Check sheet for the modelled part. Datum: model origin and axes. Units: mm. A direction names the side the tool comes from. Round coordinates to 2 decimals unless told otherwise and drop trailing zeros. Write each loop counter-clockwise with the first axis right and the second up, starting at its lowest first coordinate (ties: lowest second). Pieces come first, ordered by that corner, then holes.
Item 1: Go/stop test with flat-tipped pins: pin 1 Ø1.3 at (x, z) = (15, 39.48) entering from -Y; pin 2 Ø12 at (x, z) = (34, 28.5) entering from -Y. Record where each tip stops, or that it passes through.
Item 2: Cross-section at A-A on z = 34. Enter the section's corners in (x, y) (3 decimals), plus the area to 3 significant figures.
Item 3: Release check for a two-part mould opening along Z. For faces 5 (the flat face through (32, -3, 2.5)), 6 (the cylindrical face through (42.526, -7.986, 8.852)), 7 (the cylindrical face through (15, -8, 32)), 8 (the flat face through (49.845, -6, 39)) record: +Z half, -Z half, draft (parallel to the pull), parting line (faces both ways), or undercut.
Item 4: Cross-section at D-D on z = 16. Enter the section's corners in (x, y) (3 decimals).
Item 5: Cross-section at C-C on y = -6. Count the separate pieces of the cut face and the enclosed holes in it, plus the area to 3 significant figures.
Item 6: Material ranges on line 1 (Z direction, x = 15, y = -2.75); line 2 (Z direction, x = 37.86, y = -3.75); line 3 (Z direction, x = 30, y = -6), recorded low to high.
Item 7: Tool access check on faces 1 (the flat face through (30, -7, 41)), 2 (the flat face through (23.08, -5, 56)), 3 (the flat face through (15, -9, 6)), 4 (the cylindrical face through (39.246, -1.232, 69.065)). Record the directions out of +Z, -Z, +X, -X, +Y, -Y that give a thin tool (end or side, any length) a straight path to the whole face; none if there is none.
Item 8: Cross-section at B-B on x = 30.5. Enter the section's corners in (y, z).
from build123d import *

# Parameters (mm, degrees)
SKETCH003_W     = 45
SKETCH003_H     = 75
PAD001_DEPTH    = 7
SKETCH004_R     = 0.8
SKETCH004_R_2   = 1.25
POCKET_DEPTH    = 7
POCKET002_DEPTH = 75
SKETCH007_R     = 2
SKETCH007_R_2   = 1.25
SKETCH007_R_3   = 1.5
SKETCH007_R_4   = 0.8
PAD002_DEPTH    = 2
SKETCH008_W     = 25
SKETCH008_H     = 30
SKETCH008_R     = 1.5
POCKET003_DEPTH = 2.5
FILLET_R        = 2
SKETCH009_W     = 11.78
SKETCH009_H     = 19
SKETCH009_W_2   = 21.94
SKETCH009_H_2   = 32.99
POCKET004_DEPTH = 7


with BuildPart() as part:
    # Sketch003 → Pad001 (new body)
    with BuildSketch(Plane.XZ):
        with Locations((32.5, 40)):
            Rectangle(SKETCH003_W, SKETCH003_H)
    extrude(amount=PAD001_DEPTH)

    # Sketch004 (on Face6 of Pad001) → Pocket (cut)
    with BuildSketch(Plane.XZ.offset(7)):
        with Locations((15, 39.48)):
            Circle(SKETCH004_R)
        with Locations((15, 72.5)):
            Circle(SKETCH004_R)
        with Locations((42.94, 39.48)):
            Circle(SKETCH004_R)
        with Locations((42.94, 72.5)):
            Circle(SKETCH004_R)
        with Locations((20.08, 43.49)):
            Circle(SKETCH004_R)
        with Locations((20.08, 68.49)):
            Circle(SKETCH004_R)
        with Locations((37.86, 68.49)):
            Circle(SKETCH004_R)
        with Locations((37.86, 43.49)):
            Circle(SKETCH004_R)
        with Locations((15, 7.5)):
            Circle(SKETCH004_R_2)
        with Locations((15, 34)):
            Circle(SKETCH004_R_2)
        with Locations((44, 34)):
            Circle(SKETCH004_R_2)
        with Locations((44, 7.5)):
            Circle(SKETCH004_R_2)
    extrude(amount=-POCKET_DEPTH, mode=Mode.SUBTRACT)

    # Sketch006 (on Face6 of Pocket) → Pocket002 (cut)
    with BuildSketch(Plane(origin=(0, 0, 2.5), x_dir=(1, 0, 0), z_dir=(0, 0, -1))):
        with BuildLine():
            Line((50.994764, 2.625), (49.844764, 2.625))
            Line((49.844764, 2.625), (49.844764, 0))
            Line((49.844764, 0), (55, 0))
            Line((55, 0), (55, 7))
            Line((49.844764, 7), (55, 7))
            Line((49.844764, 4.375), (49.844764, 7))
            Line((49.844764, 4.375), (50.994764, 4.375))
            ThreePointArc((50.994764, 2.625), (54, 3.5), (50.994764, 4.375))
        make_face()
    extrude(amount=-POCKET002_DEPTH, mode=Mode.SUBTRACT)

    # Sketch007 (on Face8 of Pocket002) → Pad002 (join)
    with BuildSketch(Plane.XZ.offset(7)):
        with Locations((15, 7.5)):
            Circle(SKETCH007_R)
        with Locations((15, 7.5)):
            Circle(SKETCH007_R_2, mode=Mode.SUBTRACT)
        with Locations((15, 34)):
            Circle(SKETCH007_R)
        with Locations((15, 34)):
            Circle(SKETCH007_R_2, mode=Mode.SUBTRACT)
        with Locations((44, 7.5)):
            Circle(SKETCH007_R)
        with Locations((44, 7.5)):
            Circle(SKETCH007_R_2, mode=Mode.SUBTRACT)
        with Locations((44, 34)):
            Circle(SKETCH007_R)
        with Locations((44, 34)):
            Circle(SKETCH007_R_2, mode=Mode.SUBTRACT)
        with Locations((15, 39.48)):
            Circle(SKETCH007_R_3)
        with Locations((15, 39.48)):
            Circle(SKETCH007_R_4, mode=Mode.SUBTRACT)
        with Locations((15, 72.5)):
            Circle(SKETCH007_R_3)
        with Locations((15, 72.5)):
            Circle(SKETCH007_R_4, mode=Mode.SUBTRACT)
        with Locations((42.94, 39.48)):
            Circle(SKETCH007_R_3)
        with Locations((42.94, 39.48)):
            Circle(SKETCH007_R_4, mode=Mode.SUBTRACT)
        with Locations((42.94, 72.5)):
            Circle(SKETCH007_R_3)
        with Locations((42.94, 72.5)):
            Circle(SKETCH007_R_4, mode=Mode.SUBTRACT)
    extrude(amount=PAD002_DEPTH)

    # Sketch008 (on Face2 of Pad002) → Pocket003 (cut)
    with BuildSketch(Plane(origin=(0, 0, 0), x_dir=(1, 0, 0), z_dir=(0, 1, 0))):
        with Locations((28.97, -55.99)):
            Rectangle(SKETCH008_W, SKETCH008_H)
        with Locations((20.08, -43.49)):
            Circle(SKETCH008_R, mode=Mode.SUBTRACT)
        with Locations((37.86, -43.49)):
            Circle(SKETCH008_R, mode=Mode.SUBTRACT)
        with Locations((20.08, -68.49)):
            Circle(SKETCH008_R, mode=Mode.SUBTRACT)
        with Locations((37.86, -68.49)):
            Circle(SKETCH008_R, mode=Mode.SUBTRACT)
    extrude(amount=-POCKET003_DEPTH, mode=Mode.SUBTRACT)

    # Fillet
    fillet_edges = [part.edges().sort_by_distance(p)[0] for p in [
        (16.47, -1.25, 40.99),
        (41.47, -1.25, 40.99),
        (41.47, -1.25, 70.99),
        (16.47, -1.25, 70.99),
    ]]
    fillet(fillet_edges, radius=FILLET_R)

    # Sketch009 (on Face23 of Fillet) → Pocket004 (cut)
    with BuildSketch(Plane.XZ.offset(7)):
        with Locations((28.97, 55.99)):
            Rectangle(SKETCH009_W, SKETCH009_H)
        with Locations((28.97, 21.995)):
            Rectangle(SKETCH009_W_2, SKETCH009_H_2)
    extrude(amount=-POCKET004_DEPTH, mode=Mode.SUBTRACT)


solid = part.part
Response values:
1. pin 1: passes through
1. pin 2: stops at y = -7
2. outline: (10, -7) - (13, -7) - (13, -9) - (13.75, -9) - (13.75, 0) - (10, 0) - close; (16.25, -9) - (17, -9) - (17, -7) - (18, -7) - (18, 0) - (16.25, 0) - close; (39.94, -7) - (42, -7) - (42, -9) - (42.75, -9) - (42.75, 0) - (39.94, 0) - close; (45.25, -9) - (46, -9) - (46, -7) - (49.845, -7) - (49.845, -4.375) - (50.995, -4.375) arc R1.63 ccw (long way) to (50.995, -2.625) - (49.845, -2.625) - (49.845, 0) - (45.25, 0) - close
2. area: 106 mm2
3. face 5: -Z half
3. face 6: undercut
3. face 7: undercut
3. face 8: draft
4. outline: (10, -7) - (18, -7) - (18, 0) - (10, 0) - close; (39.94, -7) - (49.845, -7) - (49.845, -4.375) - (50.995, -4.375) arc R1.63 ccw (long way) to (50.995, -2.625) - (49.845, -2.625) - (49.845, 0) - (39.94, 0) - close
5. separate pieces: 1
5. enclosed holes: 14
5. area: 2,010 mm2
6. line 1: z = 2.5 to 6.25, 8.75 to 32.75, 35.25 to 38.68, 40.28 to 71.7, 73.3 to 77.5
6. line 2: z = 2.5 to 5.5, 38.49 to 42.69, 44.29 to 67.69, 69.29 to 77.5
6. line 3: z = 2.5 to 5.5, 38.49 to 46.49, 65.49 to 77.5
7. face 1: -Y
7. face 2: +Y, -Y
7. face 3: +Z, -Z, +X, -X, -Y
7. face 4: +Y
8. outline: (-7, 2.5) - (0, 2.5) - (0, 5.5) - (-7, 5.5) - close; (-7, 38.49) - (0, 38.49) - (0, 40.99) - (-2.5, 40.99) - (-2.5, 46.49) - (-7, 46.49) - close; (-7, 65.49) - (-2.5, 65.49) - (-2.5, 70.99) - (0, 70.99) - (0, 77.5) - (-7, 77.5) - close
